Geometry: final body of the model. Coordinates: model frame, mm. Face numbers are marked on the shaded views. A direction names the side the tool comes from. Coordinates: 2 decimals unless noted, no trailing zeros. Write each loop counter-clockwise with the first axis right and the second up, starting at its lowest first coordinate (ties: lowest second). Pieces come first, ordered by that corner, then holes. Notation, with made-up numbers: (32, 86) - (43, 86) arc R18 cw to (43, 120) - close; hole circle Ø8 at (2.25, 72). An arc over 180 degrees is marked (long way). Put each result on its own line as item: value.
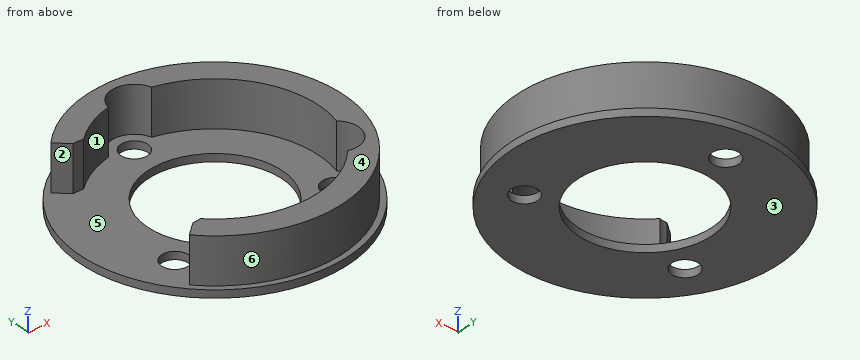
Autodesk Inventor part; units mm, degrees
ref_plane "YZ Plane" through (0, 0, 0) normal (1, 0, 0) x (0, 1, 0)
ref_plane "XZ Plane" through (0, 0, 0) normal (0, 1, 0) x (-1, 0, 0)
ref_plane "XY Plane" through (0, 0, 0) normal (0, 0, 1) x (1, 0, 0)
sketch "Sketch1" plane through (0, 0, 0) normal (0, 0, 1) x (1, 0, 0)
  circle A0 centre (0, 25) radius 3.5
  circle A1 centre (-21.6506, -12.5) radius 3.5
  circle A2 centre (21.6506, -12.5) radius 3.5
  line L0 (0, -16) -> (0, 10.5643) construction
  circle A3 centre (0, 0) radius 17.5
  circle A4 centre (0, 0) radius 35
  arc A5 (-19.6928, -15.4012) -> (19.6928, -15.4012) centre (0, 0) ccw
  arc A6 (23.1842, -9.3538) -> (3.4914, 24.755) centre (0, 0) ccw
  arc A7 (-3.4914, 24.755) -> (-23.1842, -9.3538) centre (0, 0) ccw
  dimension "d1" = 7
  dimension "d4" = 360
  dimension "d10" = 70
  dimension "d11" = 35
extrude "Extrusion1" add sketch "Sketch1" along normal blind 2 contours A0 A6 A2 A5 A1 A7 | A4
sketch "Sketch2" plane through (0, 0, 2) normal (0, 0, 1) x (1, 0, 0)
  circle A0 centre (0, 0) radius 27
  circle A1 centre (0, 0) radius 33.5
  line L0 (0, 0) -> (-23.6881, 23.6881)
  line L1 (0, 0) -> (-25.6625, -21.5334)
  line L2 (0, -27) -> (0, 12.4215) construction
  circle A2 centre (0, 25) radius 3.5
  circle A3 centre (0, 25) radius 6
  circle A4 centre (21.6506, -12.5) radius 3.5
  circle A5 centre (21.6506, -12.5) radius 6
  circle A6 centre (-21.6506, -12.5) radius 3.5
  circle A7 centre (-21.6506, -12.5) radius 6
  point P0 (-20.6832, -17.3553)
  point P1 (-19.0919, 19.0919)
  point P2 (-19.9065, -18.2409)
  point P3 (-22.0329, -18.4878)
  point P4 (-5.8438, 26.36)
  point P5 (5.8438, 26.36)
  point P6 (25.7503, -8.1191)
  point P7 (19.9065, -18.2409)
  dimension "d14" = 54
  dimension "d15" = 67
  dimension "d17" = 50
  dimension "d18" = 45
  dimension "d24" = 12
  dimension "d25" = 12
  dimension "d26" = 12
extrude "Extrusion2" add sketch "Sketch2" along normal blind 12 contours A0 A3 L0 A1 L1 A7 A5
chamfer "Chamfer1" distance 2 angle 45 1 edges at (-19.0919, 19.0919, 8)
equation "\"d19\" = d24"
properties part number "pulleycase"
1. Mould query, pull axis Y, two halves, no side actions, for the marked faces 4, 5 and 6. Classes: +Y half, -Y half, draft (parallel to the pull), parting line (faces both ways), or undercut.
Answer below:
face 4: draft
face 5: undercut
face 6: parting line
2. Ray query, probe 1 along Y at (x, z) = (0, 1.2); probe 2 along X at (y, z) = (-12.5, 1.05); probe 3 along X at (y, z) = (-15, 1). Return the intervals inside material, ascending. Write a range as from..to.
Answer below:
probe 1: y = -35..-17.5, 17.5..21.5, 28.5..35
probe 2: x = -32.69..-25.15, -18.15..-12.25, 12.25..18.15, 25.15..32.69
probe 3: x = -31.62..-24.1, -19.2..-9.01, 9.01..19.2, 24.1..31.62
3. Set-up query: the marked faces 1, 2 and 3. Return all of +Z, -Z, +X, -X, +Y, -Y with unobstructed straight access to the full face (end or side cutting, diameter ignored); none if empty.
Answer below:
face 1: +Z
face 2: +Z, -X
face 3: -Z, +X, -X, +Y, -Y
4. Section query D-D (y = -12.5). Return loops of the section in (x, z).
Answer below:
outline: (-32.69, 0) - (-25.15, 0) - (-25.15, 2) - (-32.69, 2) - close; (-18.15, 0) - (-12.25, 0) - (-12.25, 2) - (-18.15, 2) - close; (12.25, 0) - (18.15, 0) - (18.15, 2) - (12.25, 2) - close; (25.15, 0) - (32.69, 0) - (32.69, 2) - (31.08, 2) - (31.08, 14) - (27.65, 14) - (27.65, 2) - (25.15, 2) - close
5. Pin query (flat end, axial travel): pin 1 Ø1 at (y, z) = (-7, 1.5) entering from -X; pin 2 Ø6.5 at (x, y) = (21.65, -12.5) entering from -Z; pin 3 Ø1.5 at (x, y) = (-13, -17) entering from +Z; pin 4 Ø1 at (y, z) = (-11, 3.5) entering from +X. Return the tip coordinate at first contact, or that it passes through.
Answer below:
pin 1: stops at x = -34.39
pin 2: passes through
pin 3: stops at z = 2
pin 4: stops at x = 31.81
6. Section query A-A (y = 0). Return loops of the section in (x, z), then the cut area to 3 significant figures.
Answer below:
outline: (-35, 0) - (-17.5, 0) - (-17.5, 2) - (-35, 2) - close; (17.5, 0) - (35, 0) - (35, 2) - (33.5, 2) - (33.5, 14) - (27, 14) - (27, 2) - (17.5, 2) - close
area: 148 mm²
7. Section query B-B (x = 0). Return loops of the section in (y, z).
Answer below:
outline: (-35, 0) - (-17.5, 0) - (-17.5, 2) - (-27, 2) - (-27, 14) - (-33.5, 14) - (-33.5, 2) - (-35, 2) - close; (17.5, 0) - (21.5, 0) - (21.5, 2) - (17.5, 2) - close; (28.5, 0) - (35, 0) - (35, 2) - (33.5, 2) - (33.5, 14) - (31, 14) - (31, 2) - (28.5, 2) - close
8. Section query C-C (x = 13.5). Return loops of the section in (y, z).
Answer below:
outline: (-32.29, 0) - (-11.14, 0) - (-11.14, 2) - (-23.38, 2) - (-23.38, 14) - (-30.66, 14) - (-30.66, 2) - (-32.29, 2) - close; (11.14, 0) - (32.29, 0) - (32.29, 2) - (30.66, 2) - (30.66, 14) - (23.38, 14) - (23.38, 2) - (11.14, 2) - close
